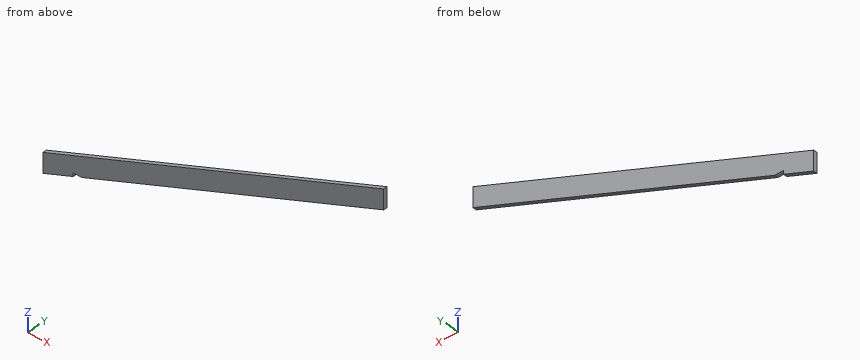
```python
from build123d import *

# Parameters (mm, degrees)
F2_DEPTH = 38.1
F3_SCALE = 0.0114810563


with BuildPart() as f2:
    # F1 (on Front) → F2 (new body)
    with BuildSketch(Plane.XZ):
        Polygon((0, 2863.85), (3048, 4083.05), (3048, 4281.3856198468), (-393.7, 2904.7056198468), (-393.7, 2706.37), (-88.9, 2828.29), (-88.9, 2863.85), align=None)
    extrude(amount=F2_DEPTH)


with BuildPart() as f2_1:
    # F3: moved
    add(f2.part.scale(F3_SCALE))


solid = f2_1.part
```
Design review of the part built by this model. Coordinates are the model's own, in mm. Give positions to 0.01 mm unless a question says otherwise; leave off trailing zeros. Write each loop counter-clockwise with the first axis right and the second up, starting at its lowest first coordinate (ties: lowest second). Pieces come first, ordered by that corner, then holes.
(1) Clearance check with a flat-ended pin moving along its axis: pin 1 Ø1.5 at (x, z) = (8, 34) entering from +Y. State where the tip first meets the part, or that it passes through.
Checked values:
pin 1: passes through
(2) Add section B-B (z = 34.5). Give the boundary of the cut face in (x, y), and give its area (3 significant figures).
Checked values:
outline: (-1.64, -0.44) - (4.05, -0.44) - (4.05, 0) - (-1.64, 0) - close
area: 2.49 mm2
(3) Add section C-C (x = 28). Give the boundary of the cut face in (y, z).
Checked values:
outline: (-0.44, 44.08) - (0, 44.08) - (0, 46.36) - (-0.44, 46.36) - close
(4) Add section A-A (y = -0.2). Give the boundary of the cut face in (x, z), and give its area (3 significant figures).
Checked values:
outline: (-4.52, 31.07) - (-1.02, 32.47) - (-1.02, 32.88) - (0, 32.88) - (34.99, 46.88) - (34.99, 49.15) - (-4.52, 33.35) - close
area: 89.8 mm2
(5) Wall thickness on line 1 along Z through (x, y) = (4, -0.3); line 2 along Z through (x, y) = (25, -0.25): over which ranges is each line inside the solid? List them lowest first.
Checked values:
line 1: z = 34.48 to 36.76
line 2: z = 42.88 to 45.16
